Part print with two shaded views. Sizes in mm from the minimum x, y, z corner. A direction names the side the tool comes from. Give positions to 0.01 mm unless a question says otherwise; leave off trailing zeros. Order: outer loops, then holes, each group sorted by start corner. A loop starts at its lowest first (then second) coordinate and runs counter-clockwise, first axis right, second up.
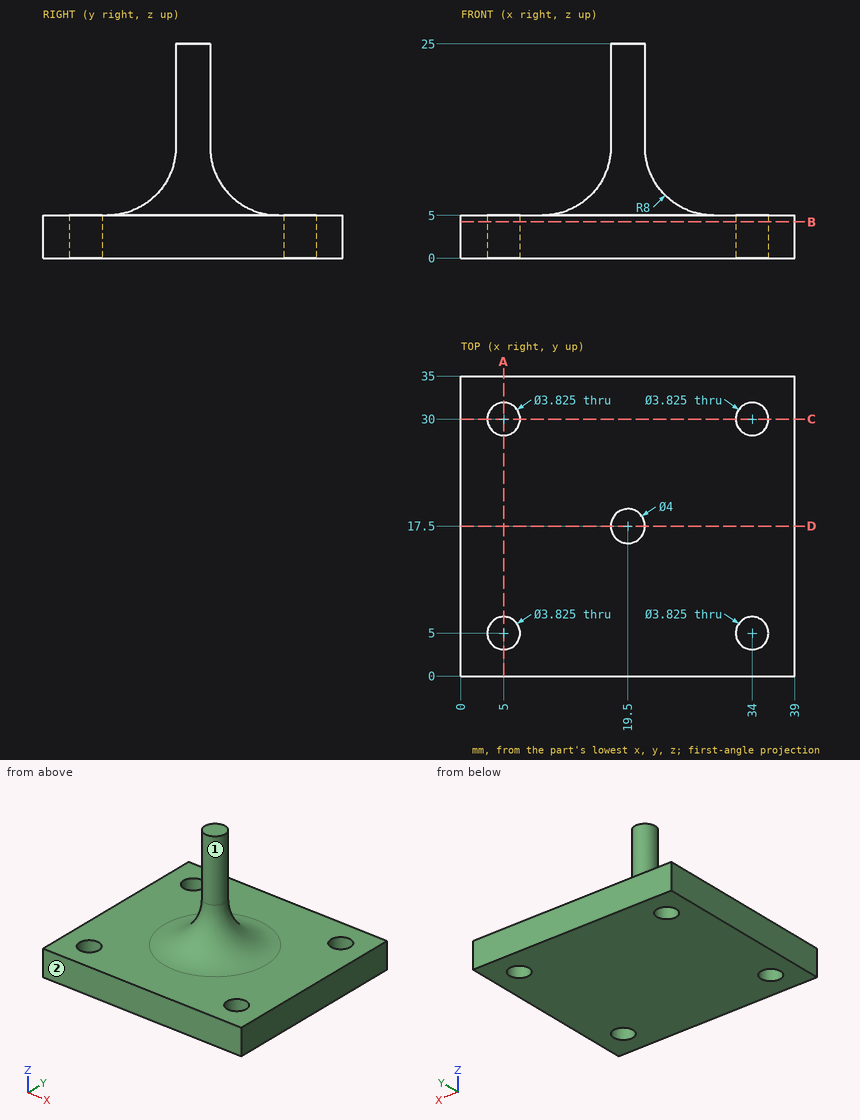
1. 3-axis set-ups, long thin cutter, end or side, ignore diameter. For the marked faces 1 and 2: which of +Z, -Z, +X, -X, +Y, -Y reach the whole face in a straight line?
2. Wall check: line 1 (Y direction, x = 5, z = 1.7); line 2 (X direction, y = 31.5, z = 4.5) (1 decimal); line 3 (Z direction, x = 33, y = 23). Give the ranges that are in metal, low to high.
3. Saw through at B-B on z = 4.25. Give the cut face in (x, y) (1 decimal).
4. Saw through at D-D on y = 17.5. Give the cut face in (x, z).
5. Saw through at A-A on x = 5. Give the cut face in (y, z), plus the area to 3 significant figures.
6. Pin check, flat tips, straight feed: P1, Ø12, axis at y = 24, z = 5.5, coming from the +X side; P2, Ø5, axis at y = 20.5, z = 18, coming from the +X side; P3, Ø10, axis at x = 8.5, y = 16, coming from the +Z side (1 decimal); P4, Ø6, axis at x = 34, y = 5, coming from the +Z side. Stop position of each tip, or through.
7. Saw through at C-C on y = 30. Give the cut face in (x, z), plus the area to 3 significant figures.
Reported:
1. face 1: +Z
1. face 2: +Z, -Z, +X, -X, -Y
2. line 1: y = 0 to 3.09, 6.91 to 28.09, 31.91 to 35
2. line 2: x = 0 to 3.8, 6.2 to 32.8, 35.2 to 39
2. line 3: z = 0 to 5
3. outline: (0, 0) - (39, 0) - (39, 35) - (0, 35) - close; hole circle Ø3.8 at (5, 5); hole circle Ø3.8 at (5, 30); hole circle Ø3.8 at (34, 5); hole circle Ø3.8 at (34, 30)
4. outline: (0, 0) - (39, 0) - (39, 5) - (29.5, 5) arc R8 cw to (21.5, 13) - (21.5, 25) - (17.5, 25) - (17.5, 13) arc R8 cw to (9.5, 5) - (0, 5) - close
5. outline: (0, 0) - (3.09, 0) - (3.09, 5) - (0, 5) - close; (6.91, 0) - (28.09, 0) - (28.09, 5) - (6.91, 5) - close; (31.91, 0) - (35, 0) - (35, 5) - (31.91, 5) - close
5. area: 137 mm2
6. P1: stops at x = 39
6. P2: stops at x = 21.44
6. P3: stops at z = 6
6. P4: stops at z = 5
7. outline: (0, 0) - (3.09, 0) - (3.09, 5) - (0, 5) - close; (6.91, 0) - (32.09, 0) - (32.09, 5) - (6.91, 5) - close; (35.91, 0) - (39, 0) - (39, 5) - (35.91, 5) - close
7. area: 157 mm2
